Read the model definition and answer for the solid it produces. Units are mm, in the model's axes. Face numbers are marked on the shaded views. A direction names the side the tool comes from. Give positions to 0.01 mm unless a question says otherwise; leave off trailing zeros. Write each loop counter-clockwise with the first axis right and the second up, starting at its lowest first coordinate (ties: lowest second). Pieces come first, ordered by that corner, then holes. Notation, with made-up numbers: M 78,83.25 L 107,83.25 A13 ccw 107,104.25 Z; hole C 69.25,-12.5 d4. An arc over 180 degrees is marked long. Answer as CSV lines item,"result". Start each with the question number.
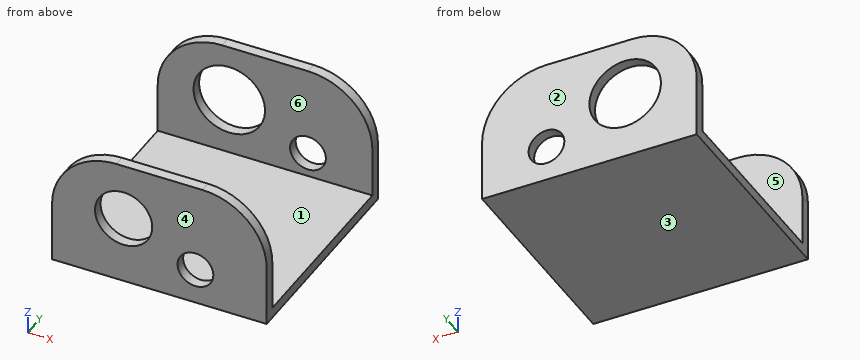
```python
from build123d import *

# Parameters (mm, degrees)
F0_W     = 30
F0_H     = 30
F1_DEPTH = 1.5
F2_W     = 30
F2_H     = 1.5
F3_DEPTH = 16
F4_W     = 30
F4_H     = 1.5
F5_DEPTH = 16
F6_R     = 4
F6_R_2   = 2.5
F7_DEPTH = 25
F8_R     = 5
F8_R_2   = 2.5
F9_DEPTH = 25
F10_R    = 9


with BuildPart() as f1:
    # F0 (on Top) → F1 (new body)
    with BuildSketch(Plane.XY):
        Rectangle(F0_W, F0_H)
    extrude(amount=F1_DEPTH)

    # F2 (on face) → F3 (join)
    with BuildSketch(Plane.XY.offset(1.5)):
        with Locations((0, 14.25)):
            Rectangle(F2_W, F2_H)
    extrude(amount=F3_DEPTH)

    # F4 (on face) → F5 (join)
    with BuildSketch(Plane.XY.offset(1.5)):
        with Locations((0, -14.25)):
            Rectangle(F4_W, F4_H)
    extrude(amount=F5_DEPTH)

    # F6 (on face) → F7 (cut)
    with BuildSketch(Plane.XZ.offset(15)):
        with Locations((-5, 9.5)):
            Circle(F6_R)
        with Locations((5.03743, 5)):
            Circle(F6_R_2)
    extrude(amount=-F7_DEPTH, mode=Mode.SUBTRACT)

    # F8 (on face) → F9 (cut)
    with BuildSketch(Plane(origin=(0, 15, 0), x_dir=(-1, 0, 0), z_dir=(0, 1, 0))):
        with Locations((5, 9.5)):
            Circle(F8_R)
        with Locations((-6, 5)):
            Circle(F8_R_2)
    extrude(amount=-F9_DEPTH, mode=Mode.SUBTRACT)

    # F10
    f10_edges = [f1.edges().sort_by_distance(p)[0] for p in [
        (15, 14.25, 17.5),
        (15, -14.25, 17.5),
        (-15, -14.25, 17.5),
        (-15, 14.25, 17.5),
    ]]
    fillet(f10_edges, radius=F10_R)


solid = f1.part
```
1. Find section A-A on z = 2. Determine the outline of the cut face in (x, y), then the cut area to 3 significant figures.
2. Given pin 1 (1 mm diameter, centred on x = 8.5, y = 10, fed in from +Z); pin 2 (3 mm diameter, centred on x = 6, z = 5, fed in from -Y), each flat-ended and moving along its own axis, determine where each tip first touches the part or whether it passes through.
3. Find section D-D on y = 12. Determine the outline of the cut face in (x, z).
4. Find section B-B on x = -5. Determine the outline of the cut face in (y, z), then the cut area to 3 significant figures.
5. For the marked faces 1 and 2, determine the directions among +Z, -Z, +X, -X, +Y, -Y from which every point of the face is accessible in a straight line to the end or side of a thin tool.
6. Determine the mould class of the marked faces 3, 4, 5 and 6 for opening direction Y: +Y half, -Y half, draft (parallel to the pull), parting line (faces both ways), or undercut.
7. Find section C-C on z = 9.5. Determine the outline of the cut face in (x, y).
8. Find the intervals of material crossed by line 1 (Y direction, x = -2, z = 14.75); line 2 (Z direction, x = -5, y = -13.8); line 3 (Z direction, x = -5, y = 14.45), in increasing order. Write a range as [from, to].
Computed:
1,outline,"M -15,-15 L 15,-15 L 15,-13.5 L -15,-13.5 Z; M -15,13.5 L 15,13.5 L 15,15 L -15,15 Z"
1,area,"90.0 mm^2"
2,pin 1,"stops at z = 1.5"
2,pin 2,"passes through"
3,outline,"M -15,0 L 15,0 L 15,1.5 L -15,1.5 Z"
4,outline,"M -15,0 L 15,0 L 15,4.5 L 13.5,4.5 L 13.5,1.5 L -13.5,1.5 L -13.5,5.5 L -15,5.5 Z; M -15,13.5 L -13.5,13.5 L -13.5,17.5 L -15,17.5 Z; M 13.5,14.5 L 15,14.5 L 15,17.5 L 13.5,17.5 Z"
4,area,"66.0 mm^2"
5,face 1,"+Z, +X, -X"
5,face 2,"+Z, -Z, +X, -X, +Y"
6,face 3,"draft"
6,face 4,"-Y half"
6,face 5,"undercut"
6,face 6,"undercut"
7,outline,"M -14.94,-15 L -9,-15 L -9,-13.5 L -14.94,-13.5 Z; M -14.94,13.5 L -10,13.5 L -10,15 L -14.94,15 Z; M -1,-15 L 14.94,-15 L 14.94,-13.5 L -1,-13.5 Z; M 0,13.5 L 14.94,13.5 L 14.94,15 L 0,15 Z"
8,line 1,"y = [-15, -13.5], [13.5, 15]"
8,line 2,"z = [0, 5.5], [13.5, 17.5]"
8,line 3,"z = [0, 4.5], [14.5, 17.5]"
